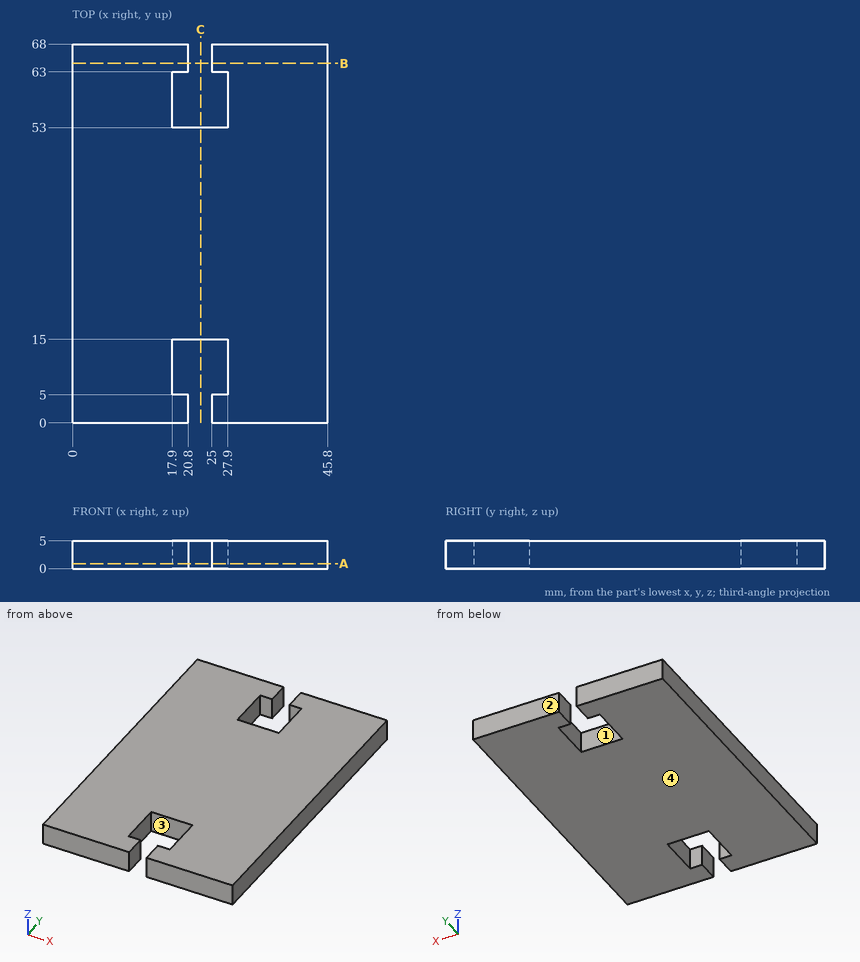
Check sheet for the drawn part. Datum: minimum x, y, z corner. Units: mm. A direction names the side the tool comes from. Give positions to 0.01 mm unless a question says otherwise; leave off trailing zeros. Order: outer loops, then holes, each group sorted by start corner. A loop starts at its lowest first (then second) coordinate and runs counter-clockwise, first axis right, second up.
1. Sectioned sample at B-B (y = 64.5). Record the boundary of the cut face in (x, z), then the cut area to 3 significant figures.
Completed:
outline: (0, 0) - (20.8, 0) - (20.8, 5) - (0, 5) - close; (25, 0) - (45.8, 0) - (45.8, 5) - (25, 5) - close
area: 208 mm2
2. Access from +Z, -Z, +X, -X, +Y, -Y to the whole of each face (thin tool, end or side, straight path). Record for the marked faces 3 and 4.
Completed:
face 3: +Z, -Z
face 4: -Z, +X, -X, +Y, -Y
3. Depth check by flat-ended pin: pin 1 (1.5 mm diameter, centred on x = 23.5, z = 2.5, fed in from +Y). Enter the tip coordinate at first touch or a pass-through.
Completed:
pin 1: stops at y = 53
4. Sectioned sample at A-A (z = 0.9). Record the boundary of the cut face in (x, y).
Completed:
outline: (0, 0) - (20.8, 0) - (20.8, 5) - (17.9, 5) - (17.9, 15) - (27.9, 15) - (27.9, 5) - (25, 5) - (25, 0) - (45.8, 0) - (45.8, 68) - (25, 68) - (25, 63) - (27.9, 63) - (27.9, 53) - (17.9, 53) - (17.9, 63) - (20.8, 63) - (20.8, 68) - (0, 68) - close
5. Draft check along X on the marked faces 1 and 2. Enter one of: pulls with the +X half, pulls with the -X half, needs draft (parallel to the pull), parting line crosses it, or undercut.
Completed:
face 1: undercut
face 2: needs draft
6. Scan lines: line 1 (Y direction, x = 27, z = 2.95); line 2 (X direction, y = 61.5, z = 0.75); line 3 (Y direction, x = 22.5, z = 0.85). Record each from-to range of solid material in increasing order.
Completed:
line 1: y = 0 to 5, 15 to 53, 63 to 68
line 2: x = 0 to 17.9, 27.9 to 45.8
line 3: y = 15 to 53
7. Sectioned sample at C-C (x = 23). Record the boundary of the cut face in (y, z).
Completed:
outline: (15, 0) - (53, 0) - (53, 5) - (15, 5) - close
